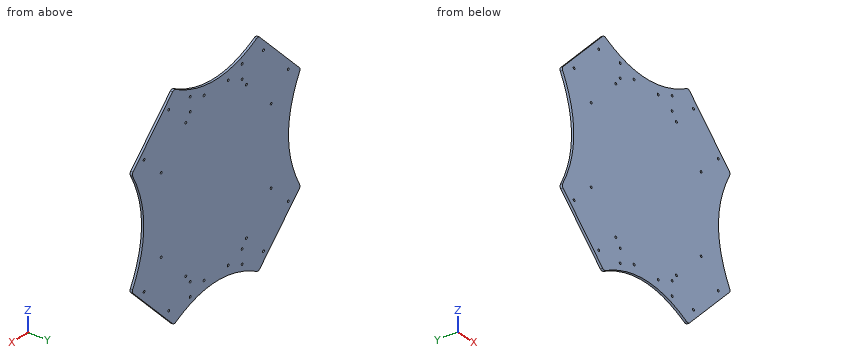
```python
from build123d import *

# Parameters (mm, degrees)
DODANIE_WYCI_GNI_CIE1_DEPTH = 3
ZAOKR_GLENIE1_R             = 4
SZKIC2_R                    = 1.5
WYTNIJ_WYCI_GNI_CIE1_DEPTH  = 197.640104054
SZYK_KO_OWY1_COUNT          = 4
SZKIC3_R                    = 1.5
WYTNIJ_WYCI_GNI_CIE2_DEPTH  = 197.640104054
SZYK_KO_OWY2_OUTLINE_R      = 1.5
SZYK_KO_OWY2_DEPTH          = 3


# Read off the part's stored shape, not the designer's step: Szyk kołowy2
with BuildPart() as part:
    # Szkic1 → Dodanie-wyciągnięcie1 (new body)
    with BuildSketch(Plane(origin=(0, 0, 0), x_dir=(1, 0, 0), z_dir=(0, 1, 0))):
        with BuildLine():
            Line((-70, -140), (-140, -70))
            add(Edge.make_bspline(
                [(-140, 70), (-100, 0), (-140, -70)],
                knots=[0, 0, 0, 1, 1, 1], degree=2))
            Line((-140, 70), (-70, 140))
            add(Edge.make_bspline(
                [(70, 140), (0, 100), (-70, 140)],
                knots=[0, 0, 0, 1, 1, 1], degree=2))
            Line((70, 140), (140, 70))
            add(Edge.make_bspline(
                [(140, -70), (100, 0), (140, 70)],
                knots=[0, 0, 0, 1, 1, 1], degree=2))
            Line((140, -70), (70, -140))
            add(Edge.make_bspline(
                [(-70, -140), (0, -100), (70, -140)],
                knots=[0, 0, 0, 1, 1, 1], degree=2))
        make_face()
    extrude(amount=DODANIE_WYCI_GNI_CIE1_DEPTH)

    # Zaokrąglenie1
    zaokr_glenie1_edges = [part.edges().sort_by_distance(p)[0] for p in [
        (-140, 1.5, -70),
        (-70, 1.5, -140),
        (70, 1.5, -140),
        (140, 1.5, -70),
        (140, 1.5, 70),
        (70, 1.5, 140),
        (-140, 1.5, 70),
        (-70, 1.5, 140),
    ]]
    fillet(zaokr_glenie1_edges, radius=ZAOKR_GLENIE1_R)

    # Szkic2 → Wytnij-wyciągnięcie1 (cut, through all)
    with BuildSketch(Plane(origin=(0, 3, 0), x_dir=(1, 0, 0), z_dir=(0, 1, 0))):
        with Locations(Location((-78.488852712, -119.501046021, 0), (0, 0, 270))):
            Circle(SZKIC2_R)
        with Locations(Location((-119.501046021, -78.488852712, 0), (0, 0, 90))):
            Circle(SZKIC2_R)
        with Locations(Location((-50.204581464, -91.216774773, 0), (0, 0, 90))):
            Circle(SZKIC2_R)
        with Locations(Location((-91.216774773, -50.204581464, 0), (0, 0, 270))):
            Circle(SZKIC2_R)
    wytnij_wyci_gni_cie1 = extrude(amount=-WYTNIJ_WYCI_GNI_CIE1_DEPTH, mode=Mode.SUBTRACT)

    # Szyk kołowy1: Wytnij-wyciągnięcie1 ×4 about axis
    szyk_ko_owy1_axis = Axis((0, 0, 0), (0, 1, 0))
    for i in range(1, SZYK_KO_OWY1_COUNT):
        add(wytnij_wyci_gni_cie1.rotate(szyk_ko_owy1_axis, i * 360 / SZYK_KO_OWY1_COUNT), mode=Mode.SUBTRACT)

    # Szkic3 → Wytnij-wyciągnięcie2 (cut, through all)
    with BuildSketch(Plane(origin=(0, 3, 0), x_dir=(1, 0, 0), z_dir=(0, 1, 0))):
        with Locations(Location((-43.1, -119, 0), (0, 0, 270))):
            Circle(SZKIC3_R)
        with Locations(Location((-20, -110, 0), (0, 0, 270))):
            Circle(SZKIC3_R)
        with Locations(Location((-43.1, -101, 0), (0, 0, 90))):
            Circle(SZKIC3_R)
    wytnij_wyci_gni_cie2 = extrude(amount=-WYTNIJ_WYCI_GNI_CIE2_DEPTH, mode=Mode.SUBTRACT)

    # Lustro1: Wytnij-wyciągnięcie2 across plane
    add(wytnij_wyci_gni_cie2.mirror(Plane(origin=(0, 0, 0), x_dir=(0, 0, 1), z_dir=(1, 0, 0))), mode=Mode.SUBTRACT)

    # Szyk kołowy2 outline → Szyk kołowy2 (cut)
    with BuildSketch(Plane(origin=(0, 0, 0), x_dir=(1, 0, 0), z_dir=(0, 1, 0))):
        with Locations((-43.1, 101)):
            Circle(SZYK_KO_OWY2_OUTLINE_R)
        with Locations((-20, 110)):
            Circle(SZYK_KO_OWY2_OUTLINE_R)
        with Locations((-43.1, 119)):
            Circle(SZYK_KO_OWY2_OUTLINE_R)
        with Locations((43.1, 119)):
            Circle(SZYK_KO_OWY2_OUTLINE_R)
        with Locations((43.1, 101)):
            Circle(SZYK_KO_OWY2_OUTLINE_R)
        with Locations((20, 110)):
            Circle(SZYK_KO_OWY2_OUTLINE_R)
    extrude(amount=SZYK_KO_OWY2_DEPTH, mode=Mode.SUBTRACT)


solid = part.part
```
Here's how the part is built. I have some questions about the finished solid (model axes, mm). Round coordinates to 2 decimals unless told otherwise and drop trailing zeros. Order: outer loops, then holes, each group sorted by start corner. A loop starts at its lowest first (then second) coordinate and runs counter-clockwise, first axis right, second up. Notation, with made-up numbers: M 1,71 L 5,71 A19 ccw 5,85 Z; hole C -28.75,36.5 d8. An arc over 180 degrees is marked long. Answer in a Markdown table with one row per item.
Item 1: Imagine slicing it at A-A, the plane x = 105. Write out the boundary of the cut face in (y, z).
A:
| item | result |
|---|---|
| outline | M 0,-105 L 3,-105 L 3,105 L 0,105 Z |
Item 2: If I drill on L1, parallel to X at y = 1.45, z = -119 (3 decimals); L2, parallel to Z at x = 90.5, y = 1.95; L3, parallel to Z at x = -69, y = 0.3, over which ranges is the centre line in solid material (lowest first)? Write a range as from..to.
A:
| item | result |
|---|---|
| L1 | x = -91..-79.903, -77.075..-44.6, -41.6..41.6, 44.6..77.075, 79.903..91 |
| L2 | z = -119.5..-51.52, -48.89..48.89, 51.52..119.5 |
| L3 | z = -139.02..139.02 |
Item 3: Imagine slicing it at C-C, the plane z = 83.5. Write out the boundary of the cut face in (x, y).
A:
| item | result |
|---|---|
| outline | M -126.5,0 L 126.5,0 L 126.5,3 L -126.5,3 Z |
Item 4: Imagine slicing it at B-B, the plane y = 1.1. State how many separate pieces and enclosed holes the cut face has, and give its area (3 significant figures).
A:
| item | result |
|---|---|
| separate pieces | 1 |
| enclosed holes | 28 |
| area | 60,900 mm2 |
Item 5: I'm going to push flat-ended pins straight in: pin 1 (1.8 mm diameter, centred on x = 43.1, z = 119, fed in from -Y); pin 2 (3.5 mm diameter, centred on x = 43.1, z = -119, fed in from -Y). Where does each tip first touch, or does it pass through?
A:
| item | result |
|---|---|
| pin 1 | passes through |
| pin 2 | stops at y = 0 |
